Verification items for the finished model (mm, model axes). A direction names the side the tool comes from. Coordinates: 2 decimals unless noted, no trailing zeros. Order: outer loops, then holes, each group sorted by start corner. A loop starts at its lowest first (then second) coordinate and runs counter-clockwise, first axis right, second up. Notation, with made-up numbers: M 8,59.25 L 18,59.25 A18 cw 18,81.25 Z; hole C 49.5,55.25 d3. An arc over 180 degrees is marked long. Write item = value, one per line.
```python
from build123d import *

# Parameters (mm, degrees)
SKETCH_1_R          = 150
EXTRUDE_1_DEPTH     = 50
CUT_EXTRUDE_START   = -25
CUT_EXTRUDE_1_DEPTH = 25
EXTRUDE_2_DEPTH     = 25
SKETCH_4_R          = 10
EXTRUDE_3_DEPTH     = 30
SKETCH_5_R          = 25.46
EXTRUDE_4_DEPTH     = 175
SKETCH_6_R          = 10
EXTRUDE_5_DEPTH     = 10


with BuildPart() as part:
    # 草图1 → 凸台-拉伸1 (new body)
    with BuildSketch(Plane(origin=(0, 0, 0), x_dir=(1, 0, 0), z_dir=(0, 1, 0))):
        with Locations(Location((0, 0, 0), (0, 0, 270))):
            Circle(SKETCH_1_R)
    extrude(amount=EXTRUDE_1_DEPTH)

    # 草图2 → 切除-拉伸1 (cut)
    with BuildSketch(Plane(origin=(0, 50, 0), x_dir=(1, 0, 0), z_dir=(0, 1, 0)).offset(CUT_EXTRUDE_START)):
        with BuildLine():
            Line((106.066017178, -106.066017178), (63.003214204, -63.003214204))
            ThreePointArc((63.003214204, -63.003214204), (59.362488155, -66.444751486), (55.534083733, -69.676219357))
            Line((55.534083733, -69.676219357), (98.758984631, -112.901120254))
            ThreePointArc((98.758984631, -112.901120254), (102.46950766, -109.544511501), (106.066017178, -106.066017178))
        make_face()
        with BuildLine():
            ThreePointArc((69.676219357, -55.534083733), (66.444751486, -59.362488155), (63.003214204, -63.003214204))
            Line((63.003214204, -63.003214204), (106.066017178, -106.066017178))
            ThreePointArc((106.066017178, -106.066017178), (109.544511501, -102.46950766), (112.901120254, -98.758984631))
            Line((112.901120254, -98.758984631), (69.676219357, -55.534083733))
        make_face()
        with BuildLine():
            Line((14.142135624, 0), (7.071067812, -7.071067812))
            Line((7.071067812, -7.071067812), (63.003214204, -63.003214204))
            ThreePointArc((63.003214204, -63.003214204), (66.444751486, -59.362488155), (69.676219357, -55.534083733))
            Line((69.676219357, -55.534083733), (14.142135624, 0))
        make_face()
        with BuildLine():
            Line((63.003214204, -63.003214204), (7.071067812, -7.071067812))
            Line((7.071067812, -7.071067812), (0, -14.142135624))
            Line((0, -14.142135624), (55.534083733, -69.676219357))
            ThreePointArc((55.534083733, -69.676219357), (59.362488155, -66.444751486), (63.003214204, -63.003214204))
        make_face()
        with BuildLine():
            Line((55.534083733, -69.676219357), (0, -14.142135624))
            Line((0, -14.142135624), (-55.534083733, -69.676219357))
            ThreePointArc((-55.534083733, -69.676219357), (0, -89.1), (55.534083733, -69.676219357))
        make_face()
        with BuildLine():
            Line((0, -14.142135624), (-7.071067812, -7.071067812))
            Line((-7.071067812, -7.071067812), (-63.003214204, -63.003214204))
            ThreePointArc((-63.003214204, -63.003214204), (-59.362488155, -66.444751486), (-55.534083733, -69.676219357))
            Line((-55.534083733, -69.676219357), (0, -14.142135624))
        make_face()
        with BuildLine():
            Line((-63.003214204, -63.003214204), (-7.071067812, -7.071067812))
            Line((-7.071067812, -7.071067812), (-14.142135624, 0))
            Line((-14.142135624, 0), (-69.676219357, -55.534083733))
            ThreePointArc((-69.676219357, -55.534083733), (-66.444751486, -59.362488155), (-63.003214204, -63.003214204))
        make_face()
        with BuildLine():
            Line((106.066017178, 106.066017178), (63.003214204, 63.003214204))
            ThreePointArc((63.003214204, 63.003214204), (66.444751486, 59.362488155), (69.676219357, 55.534083733))
            Line((69.676219357, 55.534083733), (112.901120254, 98.758984631))
            ThreePointArc((112.901120254, 98.758984631), (109.544511501, 102.46950766), (106.066017178, 106.066017178))
        make_face()
        with BuildLine():
            ThreePointArc((-55.534083733, -69.676219357), (-59.362488155, -66.444751486), (-63.003214204, -63.003214204))
            Line((-63.003214204, -63.003214204), (-106.066017178, -106.066017178))
            ThreePointArc((-106.066017178, -106.066017178), (-102.46950766, -109.544511501), (-98.758984631, -112.901120254))
            Line((-98.758984631, -112.901120254), (-55.534083733, -69.676219357))
        make_face()
        with BuildLine():
            ThreePointArc((55.534083733, 69.676219357), (59.362488155, 66.444751486), (63.003214204, 63.003214204))
            Line((63.003214204, 63.003214204), (106.066017178, 106.066017178))
            ThreePointArc((106.066017178, 106.066017178), (102.46950766, 109.544511501), (98.758984631, 112.901120254))
            Line((98.758984631, 112.901120254), (55.534083733, 69.676219357))
        make_face()
        with BuildLine():
            Line((-106.066017178, -106.066017178), (-63.003214204, -63.003214204))
            ThreePointArc((-63.003214204, -63.003214204), (-66.444751486, -59.362488155), (-69.676219357, -55.534083733))
            Line((-69.676219357, -55.534083733), (-112.901120254, -98.758984631))
            ThreePointArc((-112.901120254, -98.758984631), (-109.544511501, -102.46950766), (-106.066017178, -106.066017178))
        make_face()
        with BuildLine():
            Line((-69.676219357, -55.534083733), (-14.142135624, 0))
            Line((-14.142135624, 0), (-69.676219357, 55.534083733))
            ThreePointArc((-69.676219357, 55.534083733), (-89.1, 0), (-69.676219357, -55.534083733))
        make_face()
        with BuildLine():
            Line((-14.142135624, 0), (-7.071067812, 7.071067812))
            Line((-7.071067812, 7.071067812), (-63.003214204, 63.003214204))
            ThreePointArc((-63.003214204, 63.003214204), (-66.444751486, 59.362488155), (-69.676219357, 55.534083733))
            Line((-69.676219357, 55.534083733), (-14.142135624, 0))
        make_face()
        with BuildLine():
            Line((-63.003214204, 63.003214204), (-7.071067812, 7.071067812))
            Line((-7.071067812, 7.071067812), (0, 14.142135624))
            Line((0, 14.142135624), (-55.534083733, 69.676219357))
            ThreePointArc((-55.534083733, 69.676219357), (-59.362488155, 66.444751486), (-63.003214204, 63.003214204))
        make_face()
        Polygon((7.071067812, -7.071067812), (0, 0), (-7.071067812, -7.071067812), (0, -14.142135624), align=None)
        Polygon((-7.071067812, -7.071067812), (0, 0), (-7.071067812, 7.071067812), (-14.142135624, 0), align=None)
        Polygon((7.071067812, 7.071067812), (0, 0), (14.142135624, 0), align=None)
        Polygon((14.142135624, 0), (0, 0), (7.071067812, -7.071067812), align=None)
        Polygon((-7.071067812, 7.071067812), (0, 0), (7.071067812, 7.071067812), (0, 14.142135624), align=None)
        with BuildLine():
            Line((0, 14.142135624), (7.071067812, 7.071067812))
            Line((7.071067812, 7.071067812), (63.003214204, 63.003214204))
            ThreePointArc((63.003214204, 63.003214204), (59.362488155, 66.444751486), (55.534083733, 69.676219357))
            Line((55.534083733, 69.676219357), (0, 14.142135624))
        make_face()
        with BuildLine():
            Line((63.003214204, 63.003214204), (7.071067812, 7.071067812))
            Line((7.071067812, 7.071067812), (14.142135624, 0))
            Line((14.142135624, 0), (69.676219357, 55.534083733))
            ThreePointArc((69.676219357, 55.534083733), (66.444751486, 59.362488155), (63.003214204, 63.003214204))
        make_face()
        with BuildLine():
            ThreePointArc((-69.676219357, 55.534083733), (-66.444751486, 59.362488155), (-63.003214204, 63.003214204))
            Line((-63.003214204, 63.003214204), (-106.066017178, 106.066017178))
            ThreePointArc((-106.066017178, 106.066017178), (-109.544511501, 102.46950766), (-112.901120254, 98.758984631))
            Line((-112.901120254, 98.758984631), (-69.676219357, 55.534083733))
        make_face()
        with BuildLine():
            Line((-106.066017178, 106.066017178), (-63.003214204, 63.003214204))
            ThreePointArc((-63.003214204, 63.003214204), (-59.362488155, 66.444751486), (-55.534083733, 69.676219357))
            Line((-55.534083733, 69.676219357), (-98.758984631, 112.901120254))
            ThreePointArc((-98.758984631, 112.901120254), (-102.46950766, 109.544511501), (-106.066017178, 106.066017178))
        make_face()
        with BuildLine():
            Line((69.676219357, 55.534083733), (14.142135624, 0))
            Line((14.142135624, 0), (89.1, 0))
            ThreePointArc((89.1, 0), (84.103986662, 29.416482245), (69.676219357, 55.534083733))
        make_face()
        with BuildLine():
            Line((89.1, 0), (14.142135624, 0))
            Line((14.142135624, 0), (69.676219357, -55.534083733))
            ThreePointArc((69.676219357, -55.534083733), (84.103986662, -29.416482245), (89.1, 0))
        make_face()
        with BuildLine():
            Line((-55.534083733, 69.676219357), (0, 14.142135624))
            Line((0, 14.142135624), (55.534083733, 69.676219357))
            ThreePointArc((55.534083733, 69.676219357), (0, 89.1), (-55.534083733, 69.676219357))
        make_face()
    extrude(amount=CUT_EXTRUDE_1_DEPTH, mode=Mode.SUBTRACT)

    # 草图3 → 凸台-拉伸2 (add)
    with BuildSketch(Plane(origin=(0, 50, 0), x_dir=(1, 0, 0), z_dir=(0, 1, 0))):
        with BuildLine():
            Line((-136.715674165, -61.715674165), (-110.355339059, -35.355339059))
            ThreePointArc((-110.355339059, -35.355339059), (-125, 0), (-110.355339059, 35.355339059))
            Line((-110.355339059, 35.355339059), (-136.715674165, 61.715674165))
            ThreePointArc((-136.715674165, 61.715674165), (-150, 0), (-136.715674165, -61.715674165))
        make_face()
        with BuildLine():
            Line((35.355339059, 110.355339059), (61.715674165, 136.715674165))
            ThreePointArc((61.715674165, 136.715674165), (0, 150), (-61.715674165, 136.715674165))
            Line((-61.715674165, 136.715674165), (-35.355339059, 110.355339059))
            ThreePointArc((-35.355339059, 110.355339059), (0, 125), (35.355339059, 110.355339059))
        make_face()
        with BuildLine():
            Line((136.715674165, 61.715674165), (110.355339059, 35.355339059))
            ThreePointArc((110.355339059, 35.355339059), (121.193976626, 19.134171618), (125, 0))
            ThreePointArc((125, 0), (121.193976626, -19.134171618), (110.355339059, -35.355339059))
            Line((110.355339059, -35.355339059), (136.715674165, -61.715674165))
            ThreePointArc((136.715674165, -61.715674165), (146.641316014, -31.564607357), (150, 0))
            ThreePointArc((150, 0), (146.641316014, 31.564607357), (136.715674165, 61.715674165))
        make_face()
        with BuildLine():
            Line((61.715674165, -136.715674165), (35.355339059, -110.355339059))
            ThreePointArc((35.355339059, -110.355339059), (0, -125), (-35.355339059, -110.355339059))
            Line((-35.355339059, -110.355339059), (-61.715674165, -136.715674165))
            ThreePointArc((-61.715674165, -136.715674165), (0, -150), (61.715674165, -136.715674165))
        make_face()
    extrude(amount=EXTRUDE_2_DEPTH)

    # 草图4 → 凸台-拉伸3 (add)
    with BuildSketch(Plane.XZ):
        with Locations(Location((0, 0, 0), (0, 0, 90))):
            Circle(SKETCH_4_R)
    extrude(amount=EXTRUDE_3_DEPTH)

    # 草图5 → 凸台-拉伸4 (add)
    with BuildSketch(Plane.XZ.offset(30)):
        with Locations(Location((0, 0, 0), (0, 0, 270))):
            Circle(SKETCH_5_R)
    extrude(amount=EXTRUDE_4_DEPTH)

    # 草图6 → 凸台-拉伸5 (add)
    with BuildSketch(Plane.XZ.offset(205)):
        with Locations(Location((0, 0, 0), (0, 0, 90))):
            Circle(SKETCH_6_R)
    extrude(amount=EXTRUDE_5_DEPTH)


solid = part.part
```
Item 1: Sectioned sample at C-C, the plane y = -67. Enter the section's corners in (x, z), then the cut area to 3 significant figures.
Report:
outline = C 0,0 d50.92
area = 2,040 mm^2
Item 2: Sectioned sample at A-A, the plane x = 0. Enter the section's corners in (y, z).
Report:
outline = M -215,-10 L -205,-10 L -205,-25.46 L -30,-25.46 L -30,-10 L 0,-10 L 0,-150 L 75,-150 L 75,-125 L 50,-125 L 50,-89.1 L 25,-89.1 L 25,89.1 L 50,89.1 L 50,125 L 75,125 L 75,150 L 0,150 L 0,10 L -30,10 L -30,25.46 L -205,25.46 L -205,10 L -215,10 Z
Item 3: Scan lines: L1, parallel to Z at x = -2, y = 39.5; L2, parallel to Y at x = 20, z = 78.5; L3, parallel to Y at x = 95, z = 52. Record each from-to range of solid material in increasing order. Write a range as from..to.
Report:
L1 = -149.99..-89.08, 89.08..149.99
L2 = 0..25
L3 = 0..50
Item 4: Tool access check on faces 5 (the flat face through (49, 62, 124)), 6 (the flat face through (-103, 50, -1)), 7 (the flat face through (-48, 62, 123)), 8 (the flat face through (124, 62, -49)), 9 (the flat face through (134, 75, -1)). Record the directions out of +Z, -Z, +X, -X, +Y, -Y that give a thin tool (end or side, any length) a straight path to the whole face; none if there is none.
Report:
face_5 = +X, +Y
face_6 = +Y
face_7 = -X, +Y
face_8 = -Z, +Y
face_9 = +Z, -Z, +X, -X, +Y
Item 5: Release check for a two-part mould opening along Z. For faces 1 (the flat face through (-77.45, 37.33, 91.59)), 2 (the flat face through (0, -205, -11)), 3 (the flat face through (77.45, 37.33, -91.59)), 4 (the cylindrical face through (9.76, -209.93, -2.17)) record: pulls with the +Z half, pulls with the -Z half, needs draft (parallel to the pull), parting line crosses it, or undercut.
Report:
face_1 = undercut
face_2 = needs draft
face_3 = undercut
face_4 = parting line crosses it
Item 6: Gauge pin test, flat ends, axial feed: pin 1 (10 mm diameter, centred on x = 51.5, z = 25.5, fed in from +Y); pin 2 (5 mm diameter, centred on y = 10.5, z = -81, fed in from +X); pin 3 (20 mm diameter, centred on x = 112, z = 14, fed in from +Y). Record the tip position at first contact, or that the pin passes through.
Report:
pin_1 = 25
pin_2 = 127.82
pin_3 = 50
Item 7: Sectioned sample at D-D, the plane x = -78. Enter the section's corners in (y, z).
Report:
outline = M 0,-128.12 L 50,-128.12 L 50,-92.14 L 25,-92.14 L 25,-63.86 L 50,-63.86 L 50,-43.07 L 25,-43.07 L 25,43.07 L 50,43.07 L 50,63.86 L 25,63.86 L 25,92.14 L 50,92.14 L 50,128.12 L 0,128.12 Z
Item 8: Sectioned sample at B-B, the plane z = -81.5. Enter the section's corners in (x, y), then the cut area to 3 significant figures.
Report:
outline = M -125.93,0 L 125.93,0 L 125.93,50 L 95.64,50 L 95.64,25 L 67.36,25 L 67.36,50 L 36.01,50 L 36.01,25 L -36.01,25 L -36.01,50 L -67.36,50 L -67.36,25 L -95.64,25 L -95.64,50 L -125.93,50 Z
area = 9,380 mm^2
